Geometry check sheet. Reference: drawing and pictorial views, mm from the part's lowest x, y, z. Give positions to 0.01 mm unless a question says otherwise; leave off trailing zeros. Order: outer loops, then holes, each group sorted by start corner. A loop starts at its lowest first (then second) coordinate and runs counter-clockwise, first axis right, second up. Notation, with made-up numbers: (63, 19) - (76, 19) arc R10 cw to (76, 25) - close; hole circle Ø9 at (28.5, -34). An arc over 180 degrees is marked (long way). Answer in a Markdown table with one row per item.
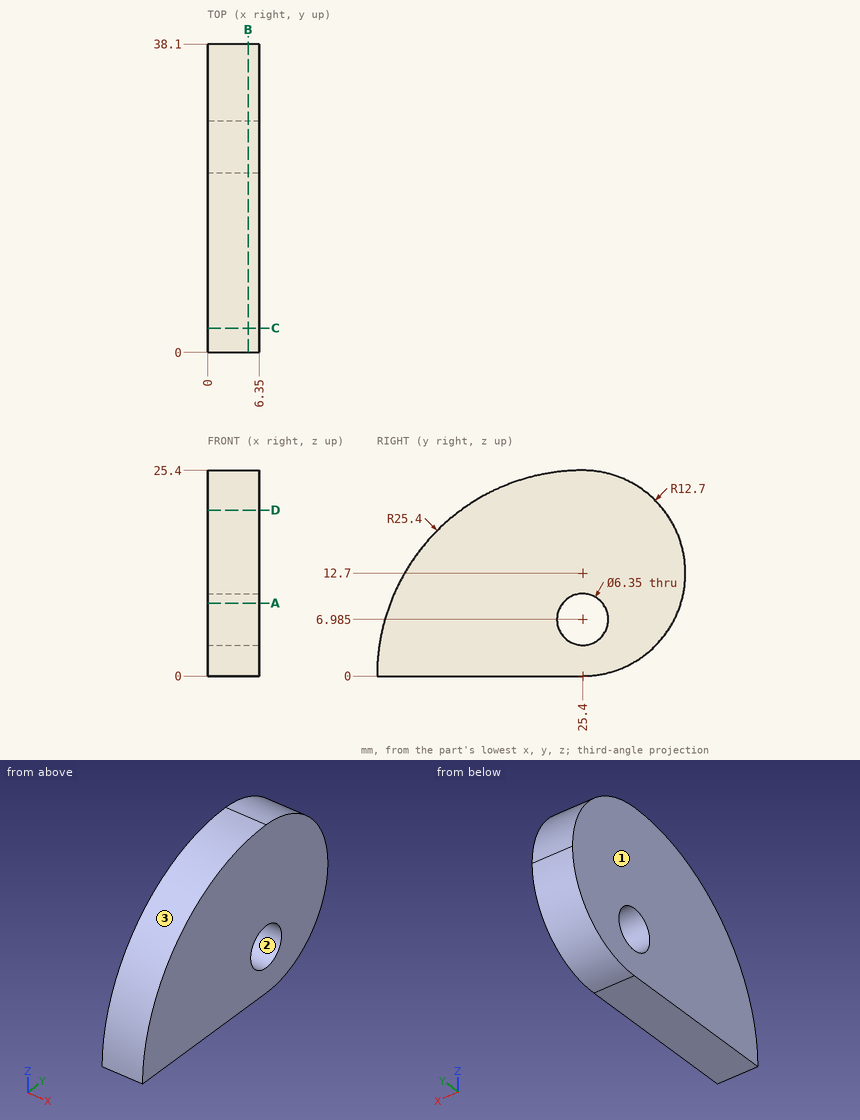
(1) Cross-section at A-A, the plane z = 9. Record the cut outline in (x, y), then the cut area to 3 significant figures.
Geometry says:
| item | result |
|---|---|
| outline | (0, 1.65) - (6.35, 1.65) - (6.35, 22.95) - (0, 22.95) - close; (0, 27.85) - (6.35, 27.85) - (6.35, 37.55) - (0, 37.55) - close |
| area | 197 mm² |
(2) Thickness scan on L1, parallel to Z at x = 3.5, y = 25.4; L2, parallel to Y at x = 3, z = 7.5; L3, parallel to Z at x = 1, y = 23. Record the ranges inside material, lowest first.
Geometry says:
| item | result |
|---|---|
| L1 | 0 to 3.81, 10.16 to 25.4 |
| L2 | 1.13 to 22.27, 28.53 to 36.99 |
| L3 | 0 to 4.91, 9.06 to 25.29 |
(3) Cross-section at C-C, the plane y = 3. Record the cut outline in (x, z).
Geometry says:
| item | result |
|---|---|
| outline | (0, 0) - (6.35, 0) - (6.35, 11.97) - (0, 11.97) - close |
(4) Cross-section at D-D, the plane z = 20.5. Record the cut outline in (x, y).
Geometry says:
| item | result |
|---|---|
| outline | (0, 10.4) - (6.35, 10.4) - (6.35, 35.42) - (0, 35.42) - close |
(5) Gauge pin test, flat end, axial feed: P1, Ø2, axis at x = 1, y = 8.5, coming from the +Z side. Record the tip position at first contact, or that the pin passes through.
Geometry says:
| item | result |
|---|---|
| P1 | z = 19.81 |
(6) Cross-section at B-B, the plane x = 5. Record the cut outline in (y, z) (3 decimals).
Geometry says:
| item | result |
|---|---|
| outline | (0, 0) - (25.4, 0) arc R12.7 ccw to (25.4, 25.4) arc R25.4 ccw to start; hole circle Ø6.35 at (25.4, 6.985) |
(7) Mould release check, pull along Y, two halves, no side actions. Record for the marked faces 1, 2 and 3: pulls with the +Y half, pulls with the -Y half, needs draft (parallel to the pull), parting line crosses it, or undercut.
Geometry says:
| item | result |
|---|---|
| face 1 | needs draft |
| face 2 | undercut |
| face 3 | pulls with the -Y half |
